```python
from build123d import *

# Parameters (mm, degrees)
EXTRUDE_THIN1_DEPTH       = 100
BOSS_EXTRUDE1_START       = -10
BOSS_EXTRUDE1_DEPTH       = 10
SKETCH3_R                 = 2.25
BOSS_EXTRUDE2_DEPTH       = 5
BOSS_EXTRUDE3_DEPTH       = 10
SKETCH5_R                 = 2.25
CUT_EXTRUDE1_DEPTH        = 6
BOSS_EXTRUDE4_REACH       = 121.416
BOSS_EXTRUDE4_END_RADIUS  = 39
SKETCH10_W                = 20
SKETCH10_H                = 20
BOSS_EXTRUDE5_START       = -39.491913729
BOSS_EXTRUDE5_OUTLINE_W   = 20
BOSS_EXTRUDE5_OUTLINE_H   = 20
BOSS_EXTRUDE5_DEPTH       = 39.491913729
BOSS_EXTRUDE5_START_2     = 91.246721786
BOSS_EXTRUDE5_2_OUTLINE_W = 23
BOSS_EXTRUDE5_2_OUTLINE_H = 23
BOSS_EXTRUDE5_2_DEPTH     = 3.753278214
BOSS_EXTRUDE6_DEPTH       = 20
SKETCH12_R                = 2.5
CUT_EXTRUDE2_DEPTH        = 20


with BuildPart() as part:
    # Sketch1 → Extrude-Thin1 (new body)
    with BuildSketch(Plane.XY):
        with BuildLine():
            ThreePointArc((-35, 0), (0, -35), (35, 0))
            Line((35, 0), (39, 0))
            ThreePointArc((39, 0), (0, -39), (-39, 0))
            Line((-39, 0), (-35, 0))
        make_face()
    extrude(amount=EXTRUDE_THIN1_DEPTH)

    # Sketch2 → Boss-Extrude1 (add)
    with BuildSketch(Plane.XY.offset(100).offset(BOSS_EXTRUDE1_START)):
        with BuildLine():
            Line((0, -39), (0, -35))
            Line((0, -35), (-10, -35))
            Line((-10, -35), (-10, -37.69615365))
            ThreePointArc((-10, -37.69615365), (-5.042321274, -38.672664715), (0, -39))
        make_face()
        with BuildLine():
            Line((10, -35), (0, -35))
            Line((0, -35), (0, -39))
            ThreePointArc((0, -39), (5.042321274, -38.672664715), (10, -37.69615365))
            Line((10, -37.69615365), (10, -35))
        make_face()
        with BuildLine():
            ThreePointArc((10, -37.69615365), (5.042321274, -38.672664715), (0, -39))
            ThreePointArc((0, -39), (-5.042321274, -38.672664715), (-10, -37.69615365))
            Line((-10, -37.69615365), (-10, -43))
            Line((-10, -43), (10, -43))
            Line((10, -43), (10, -37.69615365))
        make_face()
    extrude(amount=BOSS_EXTRUDE1_DEPTH)

    # Sketch3 → Boss-Extrude2 (add)
    with BuildSketch(Plane.XY.offset(100)):
        with Locations((-5, -39)):
            Circle(SKETCH3_R)
        with Locations((5, -39)):
            Circle(SKETCH3_R)
    extrude(amount=BOSS_EXTRUDE2_DEPTH)

    # Sketch4 → Boss-Extrude3 (add)
    with BuildSketch(Plane(origin=(0, 0, 0), x_dir=(-1, 0, 0), z_dir=(0, 0, -1))):
        with BuildLine():
            Line((0, -39), (0, -35))
            Line((0, -35), (-10, -35))
            Line((-10, -35), (-10, -37.69615365))
            ThreePointArc((-10, -37.69615365), (-5.042321274, -38.672664715), (0, -39))
        make_face()
        with BuildLine():
            ThreePointArc((10, -37.69615365), (5.042321274, -38.672664715), (0, -39))
            ThreePointArc((0, -39), (-5.042321274, -38.672664715), (-10, -37.69615365))
            Line((-10, -37.69615365), (-10, -43))
            Line((-10, -43), (10, -43))
            Line((10, -43), (10, -37.69615365))
        make_face()
        with BuildLine():
            Line((10, -35), (0, -35))
            Line((0, -35), (0, -39))
            ThreePointArc((0, -39), (5.042321274, -38.672664715), (10, -37.69615365))
            Line((10, -37.69615365), (10, -35))
        make_face()
    extrude(amount=-BOSS_EXTRUDE3_DEPTH)

    # Sketch5 → Cut-Extrude1 (cut)
    with BuildSketch(Plane(origin=(0, 0, 0), x_dir=(-1, 0, 0), z_dir=(0, 0, -1))):
        with Locations(Location((-5, -39, 0), (0, 0, 180))):
            Circle(SKETCH5_R)
        with Locations(Location((5, -39, 0), (0, 0, 180))):
            Circle(SKETCH5_R)
    extrude(amount=-CUT_EXTRUDE1_DEPTH, mode=Mode.SUBTRACT)

    # Boss-Extrude4: up to this cylinder (the profile starts outside it)
    boss_extrude4_end = Plane(origin=(0, 0, 50), z_dir=(0, 0, -1)) * Cylinder(BOSS_EXTRUDE4_END_RADIUS, 321.832, mode=Mode.PRIVATE)
    # Sketch10 → Boss-Extrude4 (add, up to the surface)
    with BuildSketch(Plane(origin=(0, -51.355775573, 4.493048169), x_dir=(1, 0, 0), z_dir=(0, 0.9961946980917462, -0.08715574274765152)), mode=Mode.PRIVATE) as boss_extrude4_sk1:
        with Locations((0, -45.680780994)):
            Rectangle(SKETCH10_W, SKETCH10_H)
    boss_extrude4_tool1 = extrude(boss_extrude4_sk1.sketch, amount=BOSS_EXTRUDE4_REACH, mode=Mode.PRIVATE) - boss_extrude4_end
    add(boss_extrude4_tool1.solids().sort_by_distance((0, -47.374433, 50))[0])

    # Boss-Extrude5: read off the stored shape, not the designer's step
    # Boss-Extrude5 outline → Boss-Extrude5 (add)
    with BuildSketch(Plane(origin=(0, -51.355775573, 4.493048169), x_dir=(1, 0, 0), z_dir=(0, 0.9961946980917462, -0.08715574274765152)).offset(BOSS_EXTRUDE5_START)):
        with Locations((0, -45.680780994)):
            Rectangle(BOSS_EXTRUDE5_OUTLINE_W, BOSS_EXTRUDE5_OUTLINE_H)
    extrude(amount=BOSS_EXTRUDE5_DEPTH)

    # Boss-Extrude5 2 outline → Boss-Extrude5 2 (cut)
    with BuildSketch(Plane(origin=(0, 0, 0), x_dir=(0.9966522374056314, 0.08110432407614805, -0.01031534248099727), z_dir=(0.08175767654690974, -0.9886876617314986, 0.12574732548071507)).offset(BOSS_EXTRUDE5_START_2)):
        with Locations((-7.5, 42.5)):
            Rectangle(BOSS_EXTRUDE5_2_OUTLINE_W, BOSS_EXTRUDE5_2_OUTLINE_H)
    extrude(amount=BOSS_EXTRUDE5_2_DEPTH, mode=Mode.SUBTRACT)

    # Sketch11 → Boss-Extrude6 (add, along a direction that is not the sketch's normal)
    with BuildSketch(Plane(origin=(10, 0, 0), x_dir=(0, 0, -1), z_dir=(1, 0, 0))):
        Polygon((-63.192356491, -83.426625408), (-43.336898209, -85.951963664), (-42.465340782, -75.990016683), (-62.320799064, -73.464678427), align=None)
    extrude(amount=BOSS_EXTRUDE6_DEPTH, dir=(0.9966471031139101, 0.0815088903864268, -0.007131103885417095))

    # Sketch12 → Cut-Extrude2 (cut)
    with BuildSketch(Plane(origin=(6.645907522, -80.368315802, 10.221732461), x_dir=(0.9966522374056314, 0.08110432407614805, -0.010315342480997362), z_dir=(-0.08175767654690974, 0.9886876617314985, -0.12574732548071624))):
        with Locations(Location((13.36525587, -47.585828212, 0), (0, 0, 270))):
            Circle(SKETCH12_R)
        with Locations(Location((13.36525587, -37.57047174, 0), (0, 0, 270))):
            Circle(SKETCH12_R)
    extrude(amount=-CUT_EXTRUDE2_DEPTH, mode=Mode.SUBTRACT)


solid = part.part
```
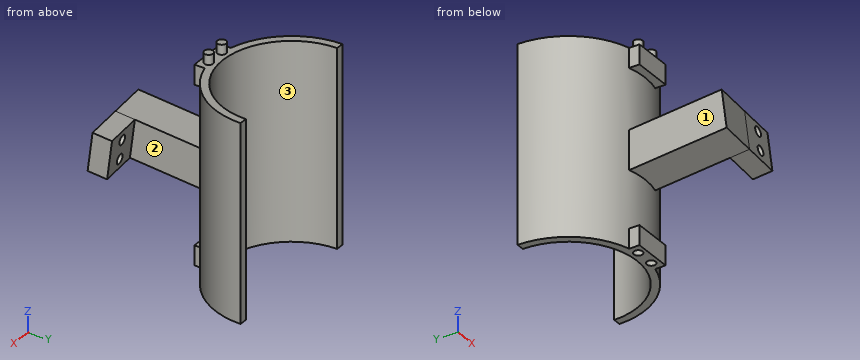
CAD build for the part. Positions are in the model's coordinates, mm. Face numbers are marked on the shaded views. Coordinates: 2 decimals unless noted, no trailing zeros. Order: outer loops, then holes, each group sorted by start corner. A loop starts at its lowest first (then second) coordinate and runs counter-clockwise, first axis right, second up. Notation, with made-up numbers: M 32.5,34 L 51.5,34 A9 ccw 51.5,50 Z; hole C 36.25,18 d5. An arc over 180 degrees is marked long. Answer as CSV lines item,"result".
1) Cut at C-C (z = 76). List the corners of the cut face in (x, y).
Verdict:
outline,"M -39,0 A39 ccw 39,0 L 35,0 A35 cw -35,0 Z"
2) Cut at D-D (x = -5). List the corners of the cut face in (y, z), then the cut area to 3 significant figures.
Verdict:
outline,"M -87.18,43.44 L -38.68,39.2 L -38.68,10 L -43,10 L -43,0 L -41.25,0 L -41.25,6 L -36.75,6 L -36.75,0 L -34.64,0 L -34.64,100 L -36.75,100 L -36.75,105 L -41.25,105 L -41.25,100 L -43,100 L -43,90 L -38.68,90 L -38.68,59.28 L -84.65,63.3 Z"
area,"1,430 mm2"
3) Cut at B-B (x = 5). List the corners of the cut face in (y, z), then the cut area to 3 significant figures.
Verdict:
outline,"M -86.36,43.37 L -38.68,39.2 L -38.68,10 L -43,10 L -43,0 L -41.25,0 L -41.25,6 L -36.75,6 L -36.75,0 L -34.64,0 L -34.64,100 L -36.75,100 L -36.75,105 L -41.25,105 L -41.25,100 L -43,100 L -43,90 L -38.68,90 L -38.68,59.28 L -83.84,63.23 Z"
area,"1,420 mm2"
4) Drill centre lines: L1, parallel to X at y = -39, z = 3; L2, parallel to Z at x = 5, y = -41; L3, parallel to X at y = -56.5, z = 56.5. Where is each one in solid material? Low to high. Write a range as from..to.
Verdict:
L1,"-10..-7.25, -2.75..2.75, 7.25..10"
L2,"6..10, 39.4..59.48, 90..105"
L3,"-10..10"
5) Cut at A-A (y = -21). List the corners of the cut face in (x, z).
Verdict:
outline,"M -32.86,0 L -28,0 L -28,100 L -32.86,100 Z; M 28,0 L 32.86,0 L 32.86,100 L 28,100 Z"
6) Mould opens along Y. For the marked faces 1, 2 and 3 say: released by +Y, released by -Y, zero draft, split by the parting line, or undercut.
Verdict:
face 1,"zero draft"
face 2,"undercut"
face 3,"released by +Y"
7) Flat gauge pins, fed straight in: P1, Ø3, axis at x = 1, z = 7.5, coming from the -Y side; P2, Ø4, axis at y = -40.5, z = 97.5, coming from the +X side; P3, Ø8, axis at x = 18.5, z = 30.5, coming from the +Y side; P4, Ø1.6, axis at x = -2, y = -39.5, coming from the -Z side. Where does each tip first touch, or does it go through?
Verdict:
P1,"y = -43"
P2,"x = 10"
P3,"y = -26.81"
P4,"z = 0"
